Source: CAD feature listing. Evaluate the final solid. Frame: model axes, mm. Round coordinates to 2 decimals unless told otherwise and drop trailing zeros. Write each loop counter-clockwise with the first axis right and the second up, starting at its lowest first coordinate (ties: lowest second). Pieces come first, ordered by that corner, then holes.
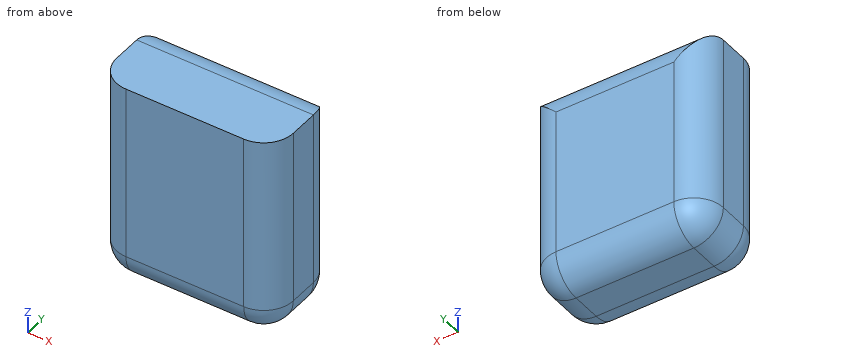
```python
from build123d import *

# Parameters (mm, degrees)
F0_W     = 30
F0_H     = 35
F1_DEPTH = 15
F2_R     = 5


with BuildPart() as f1:
    # F0 (on Front) → F1 (new body)
    with BuildSketch(Plane.XZ):
        Rectangle(F0_W, F0_H)
    extrude(amount=F1_DEPTH)

    # F2
    f2_edges = [f1.edges().sort_by_distance(p)[0] for p in [
        (0, -15, -17.5),
        (0, 0, -17.5),
        (-15, -7.5, -17.5),
        (15, -7.5, -17.5),
        (15, -15, 0),
        (-15, -15, 0),
        (15, 0, 0),
        (0, 0, 17.5),
        (-15, 0, 0),
    ]]
    fillet(f2_edges, radius=F2_R)


solid = f1.part
```
Q1. Section query A-A, the plane x = -8.5. Output: boundary loops of the cut face in (y, z), and give its area (3 significant figures).
Q2. Section query D-D, the plane x = -11.5. Output: boundary loops of the cut face in (y, z), and give its area (3 significant figures).
Q3. Line query: line 1 (Z direction, x = -12.5, y = -6.75); line 2 (Y direction, x = 11.5, z = 3); line 3 (Y direction, x = 10.75, z = -13). Output: solid intervals per line, ascending.
Q4. Pin query (flat end, axial travel): P1, Ø5, axis at y = -13, z = -1, coming from the +X side. Return the tip coordinate at first contact, or that it passes through.
Q5. Section query B-B, the plane z = -6. Output: boundary loops of the cut face in (x, y).
Q6. Section query C-C, the plane y = -3.5. Output: boundary loops of the cut face in (x, z).
Filled in:
1. outline: (-15, -12.5) arc R5 ccw to (-10, -17.5) - (-5, -17.5) arc R5 ccw to (0, -12.5) - (0, 12.5) arc R5 ccw to (-5, 17.5) - (-15, 17.5) - close
1. area: 509 mm2
2. outline: (-14.77, -12.5) arc R4.77 ccw to (-10, -17.27) - (-5, -17.27) arc R4.77 ccw to (-0.23, -12.5) - (-0.23, 14) arc R5 ccw to (-5, 17.5) - (-14.77, 17.5) - close
2. area: 491 mm2
3. line 1: z = -16.83 to 17.5
3. line 2: y = -14.77 to -0.23
3. line 3: y = -14.92 to -0.08
4. P1: stops at x = 14.97
5. outline: (-15, -10) arc R5 ccw to (-10, -15) - (10, -15) arc R5 ccw to (15, -10) - (15, -5) arc R5 ccw to (10, 0) - (-10, 0) arc R5 ccw to (-15, -5) - close
6. outline: (-14.77, -12.5) arc R4.77 ccw to (-10, -17.27) - (10, -17.27) arc R4.77 ccw to (14.77, -12.5) - (14.77, 17.27) - (-14.77, 17.27) - close
